```python
from build123d import *

# Parameters (mm, degrees)
F0_W     = 78.493316
F0_H     = 141.122394
F1_DEPTH = 7.1
F2_R     = 5.08
F3_T     = -2.54
F4_W     = 26.213542
F4_H     = 9.618692
F5_DEPTH = 12.7
F6_W     = 53.554615
F6_H     = 3.55
F6_W_2   = 4.265513
F7_DEPTH = 12.7


with BuildPart() as f1:
    # F0 (on Front) → F1 (new body)
    with BuildSketch(Plane.XZ):
        Rectangle(F0_W, F0_H)
    extrude(amount=F1_DEPTH)

    # F2
    f2_edges = [f1.edges().sort_by_distance(p)[0] for p in [
        (-39.246658, -3.55, 70.561197),
        (-39.246658, -3.55, -70.561197),
        (39.246658, -3.55, -70.561197),
        (39.246658, -3.55, 70.561197),
    ]]
    fillet(f2_edges, radius=F2_R)

    # F3
    f3_openings = [f1.faces().sort_by_distance(p)[0] for p in [
        (0, -7.1, 0),
    ]]
    offset(amount=F3_T, openings=f3_openings)

    # F4 (on face) → F5 (cut, symmetric)
    with BuildSketch(Plane.XZ.offset(2.54)):
        with Locations((23.599887, 60.043935)):
            Rectangle(F4_W, F4_H)
    extrude(amount=F5_DEPTH, both=True, mode=Mode.SUBTRACT)

    # F6 (on face) → F7 (cut, symmetric)
    with BuildSketch(Plane(origin=(0, 0, -70.561197), x_dir=(1, 0, 0), z_dir=(0, 0, -1))):
        with Locations((-7.38935, 5.325)):
            Rectangle(F6_W, F6_H)
        with Locations((21.520713, 5.325)):
            Rectangle(F6_W_2, F6_H)
    extrude(amount=F7_DEPTH, both=True, mode=Mode.SUBTRACT)


solid = f1.part
```
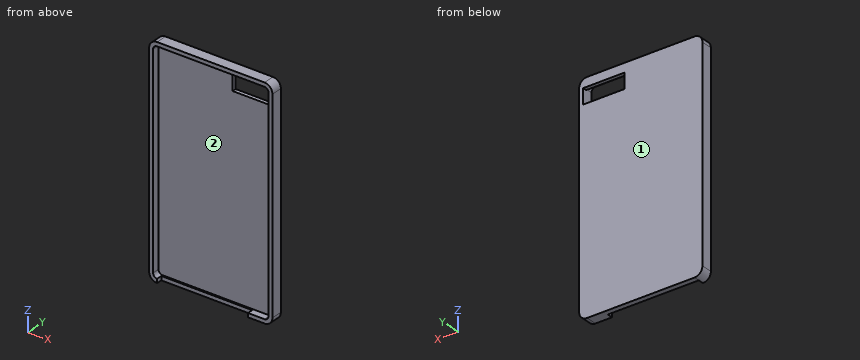
Design review of the part built by this model. Coordinates are the model's own, in mm. Face numbers are marked on the shaded views. Coordinates: 2 decimals unless noted, no trailing zeros. Loops run counter-clockwise (first coordinate to the right, second up) from the corner with the lowest first, then second, coordinate; pieces in that order, holes last. Notation, with made-up numbers: (89.25, 32.5) - (124.25, 32.5) arc R9 cw to (124.25, 44.5) - close; hole circle Ø3 at (1.25, 30.5). An arc over 180 degrees is marked (long way). Use CSV: the item, a comma, the result in double quotes. Start each with the question number.
1) Wall thickness on L1, parallel to Z at x = -25.5, y = -3.25; L2, parallel to X at y = -6.25, z = 33; L3, parallel to X at y = -1.75, z = 61.5: over which ranges is each line inside the solid? List them lowest first. Write a range as from..to.
2) Consider section B-B on z = 57. Write out the cut boundary in (x, y).
3) The part is to be moulded in two halves that separate along Z. For the marked faces 1 and 2, say which applies: +Z half, -Z half, draft (parallel to the pull), parting line (faces both ways), or undercut.
4) Consider section D-D on y = -6. Write out the cut boundary in (x, z), then the cut area to 3 significant figures.
5) Consider section A-A on x = 22. Write out the cut boundary in (y, z), then the cut area to 3 significant figures.
6) Consider section C-C on x = -11.5. Write out the cut boundary in (y, z), then the cut area to 3 significant figures.
7) For pin 1 Ø0.8 at (y, z) = (-5.5, -69.5) entering from +X; pin 2 Ø1 at (x, z) = (4, -31.5) entering from -Y; pin 3 Ø3 at (y, z) = (-5.5, -69) entering from -X, all flat-tipped, find the tip position at first contact; note any pin that passes through.
Geometry says:
1,L1,"-70.56..-68.02, 68.02..70.56"
1,L2,"-39.25..-36.71, 36.71..39.25"
1,L3,"-39.25..10.49, 36.71..39.25"
2,outline,"(-39.25, -7.1) - (-36.71, -7.1) - (-36.71, -2.54) - (10.49, -2.54) - (10.49, 0) - (-39.25, 0) - close; (36.71, -7.1) - (39.25, -7.1) - (39.25, 0) - (36.71, 0) - close"
3,face 1,"draft"
3,face 2,"undercut"
4,outline,"(-39.25, -65.48) arc R5.08 ccw to (-34.17, -70.56) - (-34.17, -68.02) arc R2.54 cw to (-36.71, -65.48) - (-36.71, 65.48) arc R2.54 cw to (-34.17, 68.02) - (34.17, 68.02) arc R2.54 cw to (36.71, 65.48) - (36.71, -65.48) arc R2.54 cw to (34.17, -68.02) - (23.65, -68.02) - (23.65, -70.56) - (34.17, -70.56) arc R5.08 ccw to (39.25, -65.48) - (39.25, 65.48) arc R5.08 ccw to (34.17, 70.56) - (-34.17, 70.56) arc R5.08 ccw to (-39.25, 65.48) - close"
4,area,"926 mm^2"
5,outline,"(-7.1, 68.02) - (-2.54, 68.02) - (-2.54, 64.85) - (0, 64.85) - (0, 70.56) - (-7.1, 70.56) - close; (-3.55, -70.56) - (0, -70.56) - (0, 55.23) - (-2.54, 55.23) - (-2.54, -68.02) - (-3.55, -68.02) - close"
5,area,"348 mm^2"
6,outline,"(-7.1, 68.02) - (-2.54, 68.02) - (-2.54, -68.02) - (-3.55, -68.02) - (-3.55, -70.56) - (0, -70.56) - (0, 70.56) - (-7.1, 70.56) - close"
6,area,"373 mm^2"
7,pin 1,"x = 37.73"
7,pin 2,"y = -2.54"
7,pin 3,"x = -38.83"
